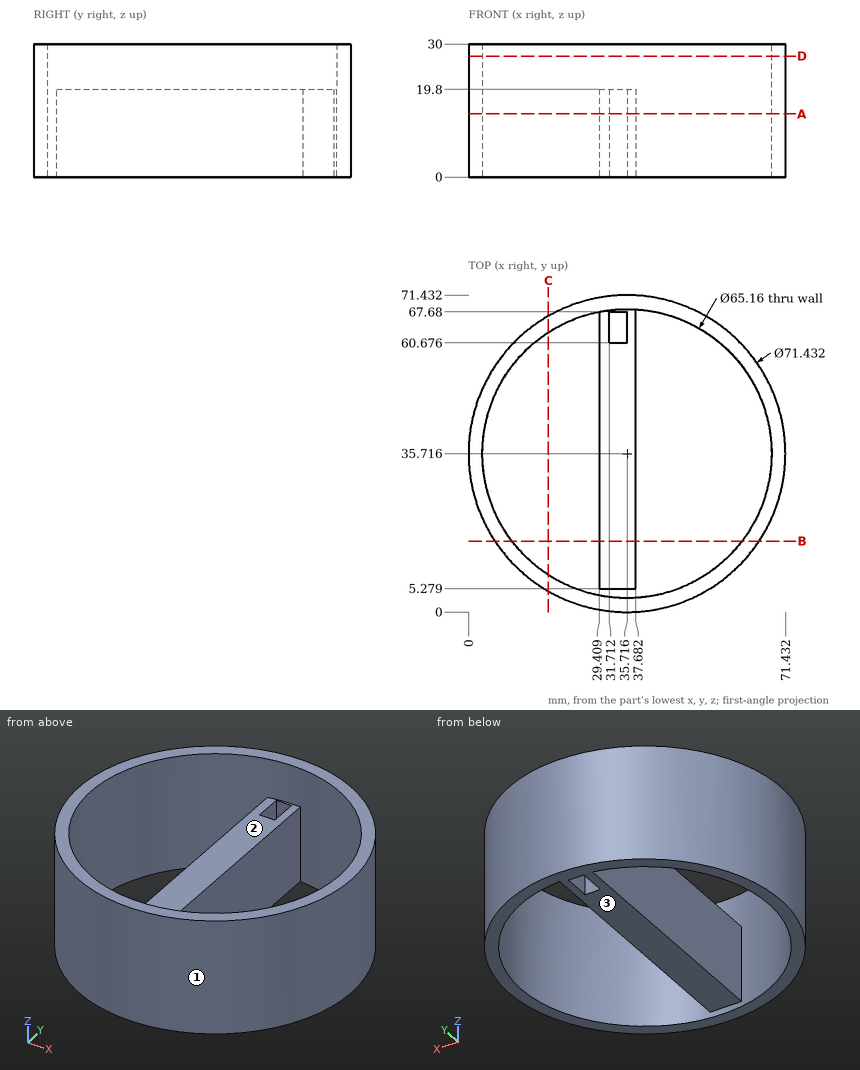
Drawing for the job (mm, zero at the part's lowest x, y, z). Give positions to 0.01 mm unless a question says otherwise; leave off trailing zeros. Loops run counter-clockwise (first coordinate to the right, second up) from the corner with the lowest first, then second, coordinate; pieces in that order, holes last.
1) Probe line 1 along X through (y, z) = (43, 5.5); line 2 along X through (y, z) = (30, 3.5); line 3 along Y through (x, z) = (17, 20.5) (1 decimal). List the from-to ranges inside material, lowest first.
Values follow:
line 1: x = 0.75 to 3.96, 29.41 to 37.68, 67.47 to 70.68
line 2: x = 0.46 to 3.64, 29.41 to 37.68, 67.79 to 70.97
line 3: y = 5.3 to 9, 62.4 to 66.1
2) Two-plate mould, pull along Y, no slides. Class the marked faces 1, 2 and 3: released by +Y, released by -Y, zero draft, split by the parting line, or undercut.
Values follow:
face 1: split by the parting line
face 2: undercut
face 3: zero draft
3) Drop flat-ended pins along their axis: P1, Ø3.5, axis at y = 66, z = 11, coming from the +X side (1 decimal); P2, Ø2, axis at x = 33.5, z = 13, coming from the +Y side; P3, Ø2, axis at x = 33, z = 10.5, coming from the -Y side; P4, Ø2, axis at x = 37, y = 8, coming from the -Z side. Give the stop position or say it passes through.
Values follow:
P1: stops at x = 57.2
P2: stops at y = 71.41
P3: stops at y = 0.04
P4: stops at z = 0
4) Band-saw the part on B-B on y = 16. List the corners of the cut face in (x, z) (1 decimal).
Values follow:
outline: (5.9, 0) - (9.8, 0) - (9.8, 30) - (5.9, 30) - close; (29.4, 0) - (37.7, 0) - (37.7, 19.8) - (29.4, 19.8) - close; (61.7, 0) - (65.5, 0) - (65.5, 30) - (61.7, 30) - close
5) Band-saw the part on D-D on z = 27.25. List the corners of the cut face in (x, y).
Values follow:
outline: circle Ø71.43 at (35.72, 35.72); hole circle Ø65.16 at (35.72, 35.72)
6) Band-saw the part on C-C on x = 18. List the corners of the cut face in (y, z), then the cut area to 3 significant figures.
Values follow:
outline: (4.7, 0) - (8.37, 0) - (8.37, 30) - (4.7, 30) - close; (63.06, 0) - (66.73, 0) - (66.73, 30) - (63.06, 30) - close
area: 220 mm2
7) Band-saw the part on A-A on z = 14.25. List the corners of the cut face in (x, y).
Values follow:
outline: circle Ø71.43 at (35.72, 35.72); hole (29.41, 5.28) - (29.41, 67.68) arc R32.58 ccw (long way) to (37.68, 68.24) - (37.68, 5.28) - close; hole (31.71, 60.68) - (35.72, 60.68) - (35.72, 67.68) - (31.71, 67.68) - close
